from build123d import *

# Parameters (mm, degrees)
F1_DEPTH = 40


with BuildPart() as f1:
    # F0 (on Front) → F1 (new body)
    with BuildSketch(Plane.XZ):
        with BuildLine():
            Line((-22.5, 0), (-15, 0))
            ThreePointArc((-15, 0), (-10.606602, 10.606602), (0, 15))
            ThreePointArc((0, 15), (10.606602, 10.606602), (15, 0))
            Line((15, 0), (22.5, 0))
            Line((22.5, 0), (22.5, 35))
            Line((22.5, 35), (7.5, 35))
            Line((7.5, 35), (7.5, 25))
            Line((7.5, 25), (-7.5, 25))
            Line((-7.5, 25), (-7.5, 35))
            Line((-7.5, 35), (-22.5, 35))
            Line((-22.5, 35), (-22.5, 0))
        make_face()
    extrude(amount=F1_DEPTH)


solid = f1.part
Check sheet for the modelled part. Datum: model origin and axes. Units: mm. A direction names the side the tool comes from. Give positions to 0.01 mm unless a question says otherwise; leave off trailing zeros. Loops run counter-clockwise (first coordinate to the right, second up) from the corner with the lowest first, then second, coordinate; pieces in that order, holes last. Notation, with made-up numbers: M 2,5 L 52,5 A26 ccw 52,43 Z; hole C 80.25,-16 d1. An arc over 180 degrees is marked long. Use a Markdown table: item, result. Add a question column.
Q1. Sectioned sample at C-C, the plane x = 12. Record the cut outline in (y, z).
Q2. Sectioned sample at A-A, the plane z = 29. Record the cut outline in (x, y), then the cut area to 3 significant figures.
Q3. Scan lines: line 1 along X through (y, z) = (-17, 30); line 2 along X through (y, z) = (-2, 11.5); line 3 along Z through (x, y) = (10.5, -14.5). Record each from-to range of solid material in increasing order. Write a range as [from, to].
Q4. Go/stop test with flat-tipped pins: pin 1 (8 mm diameter, centred on x = 3, z = 7.5, fed in from -Y); pin 2 (7.5 mm diameter, centred on x = -2.5, y = -21.5, fed in from +Z). Record where each tip stops, or that it passes through.
Q5. Mould release check, pull along X, two halves, no side actions. Record for faces 3 (the flat face through (0, -20, 25)), 4 (the flat face through (-22.5, -20, 18)), 5 (the flat face through (19, -20, 0)), 6 (the flat face through (7.5, -20, 30)): pulls with the +X half, pulls with the -X half, needs draft (parallel to the pull), parting line crosses it, or undercut.
Q6. Sectioned sample at D-D, the plane z = 6. Record the cut outline in (x, y), then the cut area to 3 significant figures.
Q7. Tool access check on faces 1 (the flat face through (-19, -20, 0)), 2 (the flat face through (-7.5, -20, 30)). Record the directions out of +Z, -Z, +X, -X, +Y, -Y that give a thin tool (end or side, any length) a straight path to the whole face; none if there is none.
Q8. Sectioned sample at B-B, the plane y = -14. Record the cut outline in (x, z), then the cut area to 3 significant figures.
Verdict:
| question | item | result |
|---|---|---|
| 1 | outline | M -40,9 L 0,9 L 0,35 L -40,35 Z |
| 2 | outline | M -22.5,-40 L -7.5,-40 L -7.5,0 L -22.5,0 Z; M 7.5,-40 L 22.5,-40 L 22.5,0 L 7.5,0 Z |
| 2 | area | 1,200 mm^2 |
| 3 | line 1 | [-22.5, -7.5], [7.5, 22.5] |
| 3 | line 2 | [-22.5, -9.63], [9.63, 22.5] |
| 3 | line 3 | [10.71, 35] |
| 4 | pin 1 | through |
| 4 | pin 2 | z = 25 |
| 5 | face 3 | undercut |
| 5 | face 4 | pulls with the -X half |
| 5 | face 5 | needs draft |
| 5 | face 6 | undercut |
| 6 | outline | M -22.5,-40 L -13.75,-40 L -13.75,0 L -22.5,0 Z; M 13.75,-40 L 22.5,-40 L 22.5,0 L 13.75,0 Z |
| 6 | area | 700 mm^2 |
| 7 | face 1 | -Z, +X, -X, +Y, -Y |
| 7 | face 2 | +Z, +Y, -Y |
| 8 | outline | M -22.5,0 L -15,0 A15 cw 0,15 A15 cw 15,0 L 22.5,0 L 22.5,35 L 7.5,35 L 7.5,25 L -7.5,25 L -7.5,35 L -22.5,35 Z |
| 8 | area | 1,070 mm^2 |
